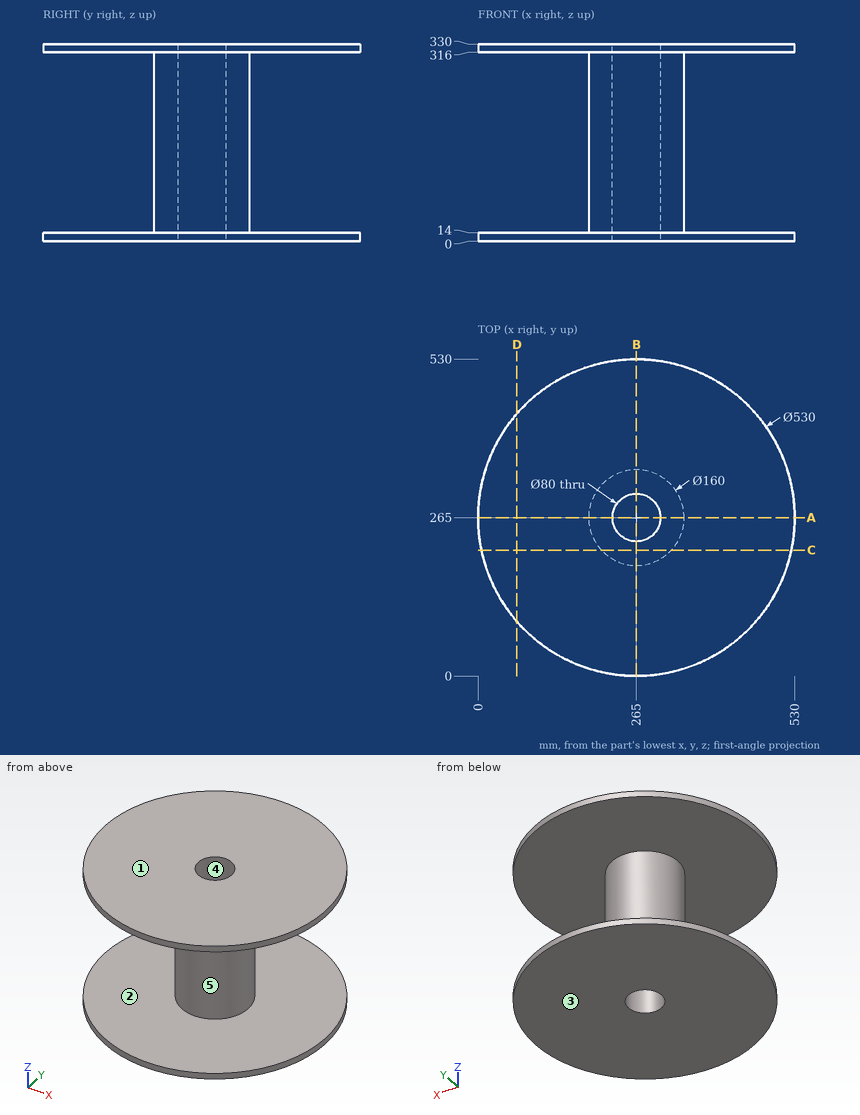
Verification items for this drawing (mm, ordinates from the low corner). A direction names the side the tool comes from. Coordinates: 2 decimals unless noted, no trailing zeros. Order: outer loops, then holes, each group sorted by start corner. A loop starts at its lowest first (then second) coordinate and runs counter-clockwise, first axis right, second up. Notation, with made-up numbers: (30, 17.5) - (76, 17.5) arc R17 cw to (76, 40.5) - close; hole circle Ø7 at (1, 55). An arc over 180 degrees is marked (long way). Answer as a JSON object with one key per item and string values. Group by question number.
Item 1: Sectioned sample at C-C, the plane y = 210.5. Record the cut outline in (x, z), and give its area (3 significant figures).
Item 2: Scan lines: probe 1 along Z at (x, y) = (98, 463); probe 2 along Y at (x, z) = (265, 148); probe 3 along Y at (x, z) = (275.5, 314). Record each from-to range of solid material in increasing order.
Item 3: Sectioned sample at A-A, the plane y = 265. Record the cut outline in (x, z), and give its area (3 significant figures).
Item 4: Draft check along Z on the marked faces 3, 4 and 5. Enter one of: +Z half, -Z half, draft (parallel to the pull), parting line (faces both ways), or undercut.
Item 5: Depth check by flat-ended pin: pin 1 Ø10 at (x, y) = (422, 407.5) entering from -Z; pin 2 Ø10 at (y, z) = (275.5, 33.5) entering from +X; pin 3 Ø3 at (x, z) = (281.5, 223) entering from +Y. Enter the tip coordinate at first touch or a pass-through.
Item 6: Sectioned sample at D-D, the plane x = 65. Record the cut outline in (y, z).
Item 7: Tool access check on the marked faces 1 and 2. Record the directions out of +Z, -Z, +X, -X, +Y, -Y that give a thin tool (end or side, any length) a straight path to the whole face; none if there is none.
Resolved:
{
 "1": {"outline": "(5.66, 0) - (524.34, 0) - (524.34, 14) - (323.56, 14) - (323.56, 316) - (524.34, 316) - (524.34, 330) - (5.66, 330) - (5.66, 316) - (206.44, 316) - (206.44, 14) - (5.66, 14) - close", "area": "49,900 mm^2"},
 "2": {"probe 1": "0 to 14, 316 to 330", "probe 2": "185 to 225, 305 to 345", "probe 3": "185.69 to 226.4, 303.6 to 344.31"},
 "3": {"outline": "(0, 0) - (225, 0) - (225, 330) - (0, 330) - (0, 316) - (185, 316) - (185, 14) - (0, 14) - close; (305, 0) - (530, 0) - (530, 14) - (345, 14) - (345, 316) - (530, 316) - (530, 330) - (305, 330) - close", "area": "36,800 mm^2"},
 "4": {"face 3": "-Z half", "face 4": "draft", "face 5": "undercut"},
 "5": {"pin 1": "z = 0", "pin 2": "x = 344.81", "pin 3": "y = 343.58"},
 "6": {"outline": "(91.15, 0) - (438.85, 0) - (438.85, 14) - (91.15, 14) - close; (91.15, 316) - (438.85, 316) - (438.85, 330) - (91.15, 330) - close"},
 "7": {"face 1": "+Z, +X, -X, +Y, -Y", "face 2": "none"}
}
